```python
from build123d import *

# Parameters (mm, degrees)
SKETCH1_W                      = 10
SKETCH1_H                      = 40
F_10_0_10_DIAMETER_HOLE1_D     = 10
F_10_0_10_DIAMETER_HOLE1_DEPTH = 40


with BuildPart() as part:
    # Sketch1 → Revolve1 (revolve)
    with BuildSketch(Plane.XZ):
        with Locations((5, 20)):
            Rectangle(SKETCH1_W, SKETCH1_H)
    revolve(axis=Axis((0, 0, 40), (0, 0, -1)))

    # Sketch2 → Revolve2 (revolve)
    with BuildSketch(Plane.XY.offset(20)):
        Polygon((20, 0), (20, 10), (15, 10), (15, 5), (8.660254038, 5), (8.660254038, 0), align=None)
    revolve(axis=Axis((8.660254038, 0, 20), (1, 0, 0)))

    # Ø10.0 (10) Diameter Hole1
    with Locations(Plane(origin=(0, 0, 0), x_dir=(-1, 0, 0), z_dir=(0, 0, -1))):
        with Locations((0, 0)):
            Hole(F_10_0_10_DIAMETER_HOLE1_D / 2, depth=F_10_0_10_DIAMETER_HOLE1_DEPTH)


solid = part.part
```
Design review of the part built by this model. Coordinates are the model's own, in mm. A direction names the side the tool comes from. Coordinates: 2 decimals unless noted, no trailing zeros. Order: outer loops, then holes, each group sorted by start corner. A loop starts at its lowest first (then second) coordinate and runs counter-clockwise, first axis right, second up.
1) Take a section at A-A, the plane x = 0. Give the boundary of the cut face in (y, z).
2) Take a section at D-D, the plane z = 20. Give the boundary of the cut face in (x, y), and give its area (3 significant figures).
3) Clearance check with flat-ended pins moving along their axes: pin 1 (4 mm diameter, centred on x = -5, z = 15, fed in from +Y); pin 2 (1.5 mm diameter, centred on y = 3, z = 32.5, fed in from -X); pin 3 (1 mm diameter, centred on x = 8, z = 15.5, fed in from +Y). State where each tip first meets the part, or that it passes through.
4) Take a section at C-C, the plane y = 0. Give the boundary of the cut face in (x, z), and give its area (3 significant figures).
5) Wall thickness on line 1 along Y through (x, z) = (0, 31); line 2 along X through (y, z) = (-1.5, 7); line 3 along Y through (x, z) = (-4.5, 3.5): over which ranges is each line inside the solid? List them lowest first.
6) Mouldability with a two-part tool opening along X and no side actions: class faces 1 (the flat face through (20, 0, 20)), 2 (the flat face through (15, -5, 18)), 3 (the cylindrical face through (17.465, -1.302, 29.915)) as +X half, -X half, draft (parallel to the pull), parting line (faces both ways), or undercut.
7) For faces 4 (the cylindrical face through (-1.08, -4.88, 20.28)), 5 (the cylindrical face through (12, 3, 24)), list the 3-axis set-ups (+Z, -Z, +X, -X, +Y, -Y) from which the entire face can be reached by the end or side of a thin tool; tool diameter is ignored.
8) Take a section at B-B, the plane z = 12.5. Give the boundary of the cut face in (x, y), and give its area (3 significant figures).
Returned:
1. outline: (-10, 0) - (-5, 0) - (-5, 40) - (-10, 40) - close; (5, 0) - (10, 0) - (10, 40) - (5, 40) - close
2. outline: (8.66, -5) - (15, -5) - (15, -10) - (20, -10) - (20, 10) - (15, 10) - (15, 5) - (8.66, 5) arc R10 ccw (long way) to start; hole circle Ø10 at (0, 0)
2. area: 390 mm2
3. pin 1: stops at y = 9.54
3. pin 2: stops at x = -9.74
3. pin 3: stops at y = 6.61
4. outline: (-10, 0) - (-5, 0) - (-5, 40) - (-10, 40) - close; (5, 0) - (10, 0) - (10, 15) - (15, 15) - (15, 10) - (20, 10) - (20, 30) - (15, 30) - (15, 25) - (10, 25) - (10, 40) - (5, 40) - close
4. area: 550 mm2
5. line 1: y = -10 to -5, 5 to 10
5. line 2: x = -9.89 to -4.77, 4.77 to 9.89
5. line 3: y = -8.93 to -2.18, 2.18 to 8.93
6. face 1: +X half
6. face 2: undercut
6. face 3: draft
7. face 4: +Z, -Z
7. face 5: none
8. outline: circle Ø20 at (0, 0); (15, -6.61) - (20, -6.61) - (20, 6.61) - (15, 6.61) - close; hole circle Ø10 at (0, 0)
8. area: 302 mm2
